The listing builds one solid part. Answer for the finished solid, in the listing's coordinates (mm). A direction names the side the tool comes from. Give positions to 0.01 mm unless a question says otherwise; leave off trailing zeros. Write each loop counter-clockwise with the first axis right and the second up, starting at its lowest first coordinate (ties: lowest second). Pieces come first, ordered by that corner, then holes. Notation, with made-up numbers: (86.5, 8.5) - (107.5, 8.5) arc R33 cw to (107.5, 38.5) - close; hole circle Ø11 at (72.25, 0.25). An arc over 180 degrees is marked (long way). Answer in a Markdown table with one row per item. Add a question column.
from build123d import *

# Parameters (mm, degrees)
SKETCH1_R           = 3.5
BOSS_EXTRUDE1_DEPTH = 48
SKETCH2_R           = 7.5
BOSS_EXTRUDE2_DEPTH = 3
CHAMFER1_SIZE       = 1
FILLET1_R           = 0.2


with BuildPart() as part:
    # Sketch1 → Boss-Extrude1 (new body)
    with BuildSketch(Plane.XY):
        Circle(SKETCH1_R)
    extrude(amount=BOSS_EXTRUDE1_DEPTH)

    # Sketch2 → Boss-Extrude2 (add)
    with BuildSketch(Plane(origin=(0, 0, 0), x_dir=(-1, 0, 0), z_dir=(0, 0, -1))):
        Circle(SKETCH2_R)
    extrude(amount=BOSS_EXTRUDE2_DEPTH)

    # Chamfer1
    chamfer1_edges = [part.edges().sort_by_distance(p)[0] for p in [
        (-3.5, 0, 48),
    ]]
    chamfer(chamfer1_edges, length=CHAMFER1_SIZE)

    # Fillet1
    fillet1_edges = [part.edges().sort_by_distance(p)[0] for p in [
        (-3.5, 0, 0),
    ]]
    fillet(fillet1_edges, radius=FILLET1_R)


solid = part.part
1. Given pin 1 Ø1 at (x, y) = (-5.5, 2.5) entering from +Z; pin 2 Ø5 at (x, y) = (1.5, -5) entering from +Z; pin 3 Ø4 at (y, z) = (3, 17) entering from +X, each flat-ended and moving along its own axis, determine where each tip first touches the part or whether it passes through.
2. Section D-D (y = 5.5) is taken. Give the vertices of the cut face in (x, z).
3. Section A-A (y = 0) is taken. Give the vertices of the cut face in (x, z), and give its area (3 significant figures).
4. Section C-C (z = 11) is taken. Give the vertices of the cut face in (x, y).
5. Straight lines are drawn through the part: L1, parallel to Z at x = 4.75, y = -4; L2, parallel to X at y = -0.75, z = 34; L3, parallel to X at y = -0.5, z = 22. For each, find the intervals that lie inside material, in ascending order. Write a range as [from, to].
6. A tool of negligible diameter and unlimited length cuts with its end or side. For faces 1 (the face through (1.77, 3.44, 0)), 2 (the face through (0, 0, -3)), from which of +Z, -Z, +X, -X, +Y, -Y can it reach the whole face along a straight path? Write none if from no direction.
Geometry check:
| question | item | result |
|---|---|---|
| 1 | pin 1 | z = 0 |
| 1 | pin 2 | z = 47.78 |
| 1 | pin 3 | x = 3.35 |
| 2 | outline | (-5.1, -3) - (5.1, -3) - (5.1, 0) - (-5.1, 0) - close |
| 3 | outline | (-7.5, -3) - (7.5, -3) - (7.5, 0) - (3.7, 0) arc R0.2 cw to (3.5, 0.2) - (3.5, 47) - (2.5, 48) - (-2.5, 48) - (-3.5, 47) - (-3.5, 0.2) arc R0.2 cw to (-3.7, 0) - (-7.5, 0) - close |
| 3 | area | 380 mm² |
| 4 | outline | circle Ø7 at (0, 0) |
| 5 | L1 | [-3, 0] |
| 5 | L2 | [-3.42, 3.42] |
| 5 | L3 | [-3.46, 3.46] |
| 6 | face 1 | +Z |
| 6 | face 2 | -Z, +X, -X, +Y, -Y |
